Can you work these out from the model? Positions are in its coordinate system, mm. Round coordinates to 2 decimals unless told otherwise and drop trailing zeros. Write each loop counter-clockwise with the first axis right and the second up, starting at its lowest first coordinate (ties: lowest second). Pieces come first, ordered by that corner, then holes. Notation, with made-up numbers: (45.5, 53.25) -> (49.5, 53.25) arc R10 ccw to (49.5, 65.25) -> close; hole circle Ø2 at (87.5, 2). An arc over 180 degrees is marked (long way). Use CSV: the item, a comma, the result in double quotes.
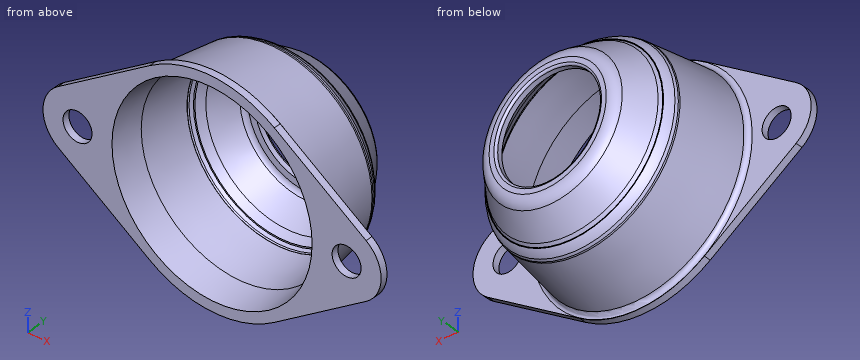
```python
from build123d import *

# Parameters (mm, degrees)
R_VOL_MINCE1_OUTLINE_W   = 0.007571627
R_VOL_MINCE1_OUTLINE_H   = 0.3920495
R_VOL_MINCE1_OUTLINE_W_2 = 0.976658528
R_VOL_MINCE1_OUTLINE_H_2 = 0.231591764
ESQUISSE2_R              = 2.1
ESQUISSE2_R_2            = 14.5
BOSS_EXTRU_1_DEPTH       = 1
CONG_1_R                 = 0.7
CONG_2_R                 = 0.3


# Read off the part's stored shape, not the designer's step: Révol.-Mince1
with BuildPart() as part:
    # Révol.-Mince1 outline → Révol.-Mince1 (revolve)
    with BuildSketch(Plane.XY):
        with BuildLine():
            Line((7.5, 17), (7.5, 16))
            Line((7.5, 16), (8.491270905, 16))
            ThreePointArc((8.491270905, 16), (8.94469782, 15.89129346), (9.299543794, 15.588808065))
            Line((9.299543794, 15.588808065), (11.571523179, 12.47))
            Line((11.571523179, 12.47), (12.5, 12.47))
            Line((12.5, 12.47), (12.5, 12.893800849))
            Line((12.5, 12.893800849), (10.107816683, 16.177616129))
            ThreePointArc((10.107816683, 16.177616129), (9.398124736, 16.782586921), (8.491270905, 17))
            Line((8.491270905, 17), (7.5, 17))
        make_face()
        Polygon((12.5, 12.47), (11.571523179, 12.47), (12.3, 11.47), (12.5, 11.47), align=None)
        Polygon((12.5, 12.893800849), (12.5, 12.47), (12.808729095, 12.47), align=None)
        Polygon((12.808729095, 12.47), (12.5, 12.47), (12.5, 11.47), (12.892428373, 11.47), (12.892428373, 12.47), align=None)
        with BuildLine():
            Line((12.892428373, 11.47), (12.5, 11.47))
            add(Edge.make_bspline(
                [(12.801834176, 11.0779505), (12.686238359, 11.297221706), (12.5, 11.47)],
                knots=[0.333971607, 0.333971607, 0.333971607, 1, 1, 1], degree=2))
            Line((12.801834176, 11.0779505), (12.892428373, 11.0779505))
            Line((12.892428373, 11.0779505), (12.892428373, 11.47))
        make_face()
        with BuildLine():
            add(Edge.make_bspline(
                [(12.9, 12.462975599), (12.897476124, 12.465317066), (12.894952248, 12.467658533), (12.892428373, 12.47)],
                knots=[0.991680034, 0.991680034, 0.991680034, 0.991680034, 1, 1, 1, 1], degree=3))
            Line((12.892428373, 12.47), (12.892428373, 11.47))
            Line((12.892428373, 11.47), (12.9, 11.47))
            Line((12.9, 11.47), (12.9, 12.462975599))
        make_face()
        with BuildLine():
            Line((12.892428373, 11.0779505), (12.801834176, 11.0779505))
            add(Edge.make_bspline(
                [(12.892428373, 10.868711363), (12.854448818, 10.978146923), (12.801834176, 11.0779505)],
                knots=[0.030821836, 0.030821836, 0.030821836, 0.333971607, 0.333971607, 0.333971607], degree=2))
            Line((12.892428373, 10.868711363), (12.892428373, 11.0779505))
        make_face()
        with Locations((12.896214186, 11.27397525)):
            Rectangle(R_VOL_MINCE1_OUTLINE_W, R_VOL_MINCE1_OUTLINE_H)
        with BuildLine():
            add(Edge.make_bspline(
                [(13.724014392, 11.47), (13.719202707, 11.479925565), (13.714323748, 11.489820846), (13.633178057, 11.651645326), (13.540873317, 11.796040705), (13.381756728, 11.995490826), (13.325317424, 12.059137243), (13.251089091, 12.134794608), (13.228544986, 12.15720053), (13.205604181, 12.179163391), (13.190224008, 12.19370632), (13.181560449, 12.201764459), (13.157861099, 12.223750978), (13.065587572, 12.309355591), (12.973314046, 12.394960203), (12.9, 12.462975599)],
                knots=[0.233772362, 0.233772362, 0.233772362, 0.233772362, 0.25, 0.25, 0.5, 0.5, 0.625, 0.625, 0.65625, 0.671875, 0.671875, 0.6875, 0.6875, 0.75, 0.991680034, 0.991680034, 0.991680034, 0.991680034], degree=3))
            Line((12.9, 12.462975599), (12.9, 11.47))
            Line((12.9, 11.47), (13.724014392, 11.47))
        make_face()
        with BuildLine():
            Line((12.892428373, 11.0779505), (12.892428373, 10.868711363))
            add(Edge.make_bspline(
                [(12.9, 10.846358736), (12.896289829, 10.857584833), (12.892428373, 10.868711363)],
                knots=[0, 0, 0, 0.030821836, 0.030821836, 0.030821836], degree=2))
            Line((12.9, 10.846358736), (12.9, 11.0779505))
            Line((12.9, 11.0779505), (12.892428373, 11.0779505))
        make_face()
        with BuildLine():
            Line((13.724014392, 11.47), (12.9, 11.47))
            Line((12.9, 11.47), (12.9, 11.0779505))
            Line((12.9, 11.0779505), (13.876658528, 11.0779505))
            add(Edge.make_bspline(
                [(13.876658528, 11.0779505), (13.868496738, 11.102646143), (13.860334948, 11.127341786), (13.848092262, 11.16438525), (13.840518996, 11.18708214), (13.82647434, 11.226996021), (13.819202463, 11.246876541), (13.785496409, 11.335579036), (13.756266672, 11.40346985), (13.724014392, 11.47)],
                knots=[0, 0, 0, 0, 0.0625, 0.0625, 0.09375, 0.09375, 0.125, 0.125, 0.233772362, 0.233772362, 0.233772362, 0.233772362], degree=3))
        make_face()
        Polygon((13.876658528, 10.846358736), (12.9, 10.846358736), (13.876658528, 4.225615763), align=None)
        with Locations((13.388329264, 10.962154618)):
            Rectangle(R_VOL_MINCE1_OUTLINE_W_2, R_VOL_MINCE1_OUTLINE_H_2)
        Polygon((13.910821774, 10.846358736), (13.876658528, 11.0779505), (13.876658528, 10.846358736), align=None)
        Polygon((13.876658528, 10.846358736), (13.876658528, 4.225615763), (14.5, 0), (15.489294083, 0.145935661), (13.910821774, 10.846358736), align=None)
    revolve(axis=Axis((0, 0, 0), (0, 1, 0)))

    # Esquisse2 → Boss.-Extru.1 (add)
    with BuildSketch(Plane(origin=(0, 0, 0), x_dir=(1, 0, 0), z_dir=(0, 1, 0))):
        with BuildLine():
            Line((-22.320512821, 4.128523638), (-9.025641026, 13.211275642))
            ThreePointArc((-9.025641026, 13.211275642), (0, 16), (9.025641026, 13.211275642))
            Line((9.025641026, 13.211275642), (22.320512821, 4.128523638))
            ThreePointArc((22.320512821, 4.128523638), (24.5, 0), (22.320512821, -4.128523638))
            Line((22.320512821, -4.128523638), (9.025641026, -13.211275642))
            ThreePointArc((9.025641026, -13.211275642), (0, -16), (-9.025641026, -13.211275642))
            Line((-9.025641026, -13.211275642), (-22.320512821, -4.128523638))
            ThreePointArc((-22.320512821, -4.128523638), (-24.5, 0), (-22.320512821, 4.128523638))
        make_face()
        with Locations(Location((-19.5, 0, 0), (0, 0, 270))):
            Circle(ESQUISSE2_R, mode=Mode.SUBTRACT)
        with Locations(Location((19.5, 0, 0), (0, 0, 90))):
            Circle(ESQUISSE2_R, mode=Mode.SUBTRACT)
        Circle(ESQUISSE2_R_2, mode=Mode.SUBTRACT)
    extrude(amount=BOSS_EXTRU_1_DEPTH)

    # Congé1
    cong_1_edges = [part.edges().sort_by_distance(p)[0] for p in [
        (-15.36330683, 1, 0),
    ]]
    fillet(cong_1_edges, radius=CONG_1_R)

    # Congé2
    cong_2_edges = [part.edges().sort_by_distance(p)[0] for p in [
        (-7.5, 17, 0),
    ]]
    fillet(cong_2_edges, radius=CONG_2_R)


solid = part.part
```
Q1. Suppose I cut it at A-A (x = -18). Write out the boundary of the cut face in (y, z), and give its area (3 significant figures).
Resolved:
outline,"(0, -7.08) -> (1, -7.08) -> (1, -1.47) -> (0, -1.47) -> close; (0, 1.47) -> (1, 1.47) -> (1, 7.08) -> (0, 7.08) -> close"
area,"11.2 mm^2"
Q2. Please list where these lines run through material, in increasing order: probe 1 along Z at (x, y) = (11.5, 2.5); probe 2 along Z at (x, y) = (-10, 10.25); probe 3 along X at (y, z) = (1.5, 2).
Resolved:
probe 1,"z = -9.85 to -8.21, 8.21 to 9.85"
probe 2,"z = -9.8 to -8.29, 8.29 to 9.8"
probe 3,"x = -15.17 to -14.14, 14.14 to 15.17"
Q3. Suppose I cut it at C-C (z = 1). Count the separate pieces of the cut face and the enclosed holes in it, and give its area (3 significant figures).
Resolved:
separate pieces,"4"
enclosed holes,"0"
area,"50.3 mm^2"
Q4. Suppose I cut it at B-B (x = 19.5). Write out the boundary of the cut face in (y, z).
Resolved:
outline,"(0, -6.06) -> (1, -6.06) -> (1, -2.1) -> (0, -2.1) -> close; (0, 2.1) -> (1, 2.1) -> (1, 6.06) -> (0, 6.06) -> close"
Q5. Will these pins go through, and if not, where does the flat tip stop? P1, Ø5, axis at y = 3, z = 4.5, coming from the +X side; P2, Ø6, axis at x = -16.5, z = 1.5, coming from the +Y side (3 decimals); P3, Ø1.5, axis at x = 3.5, y = 14.5, coming from the +Z side.
Resolved:
P1,"stops at x = 23.5"
P2,"stops at y = 11.745"
P3,"stops at z = 11.39"
